Autodesk Inventor part; units mm, degrees
ref_plane "Work Plane1" through (2.381, -7.4919, 0) normal (0, 0, -1) x (0, 1, 0)
ref_plane "Work Plane2" through (2.381, -7.4919, 0) normal (1, 0, 0) x (0, 1, 0)
ref_plane "YZ Plane" through (0, 0, 0) normal (1, 0, 0) x (0, 1, 0)
sketch "Sketch1" plane through (0, 0, 0) normal (0, 0, 1) x (1, 0, 0)
  line L0 (2.381, 29.408) -> (2.381, -22.2008)
  line L1 (-18.8276, 20.7851) -> (-24.5938, 20.7851)
  line L2 (-24.5938, 20.7851) -> (-24.5938, 18.3721)
  line L3 (-24.5938, 18.3721) -> (-23.654, 18.3721)
  line L4 (-23.654, 18.3721) -> (-23.654, 16.9751)
  line L5 (-23.654, 16.9751) -> (-24.5938, 16.9751)
  line L6 (-24.5938, 16.9751) -> (-24.5938, 14.4351)
  line L7 (-24.5938, 14.4351) -> (-23.1968, 14.4351)
  line L8 (-23.1968, 14.4351) -> (-23.1968, 12.1491)
  line L9 (-23.1968, 12.1491) -> (-24.5938, 12.1491)
  line L10 (-24.5938, 12.1491) -> (-24.5938, 10.6251)
  line L11 (-24.5938, 10.6251) -> (-23.8268, 10.6251)
  line L12 (-22.2393, 9.0376) -> (-22.2393, 1.6716)
  line L13 (-23.8268, 0.0841) -> (-25.3635, 0.0841)
  line L14 (-25.3635, 0.0841) -> (-25.3635, -2.0749)
  line L15 (-25.3635, -2.0749) -> (-23.9919, -2.0749)
  line L16 (-23.9919, -2.0749) -> (-23.9919, -4.3609)
  line L17 (-23.9919, -4.3609) -> (-25.3635, -4.3609)
  line L18 (-25.3635, -4.3609) -> (-25.3635, -7.8153)
  line L19 (-25.3635, -7.8153) -> (-26.7351, -7.8153)
  line L20 (-27.7511, -8.8313) -> (-27.7511, -13.1493)
  line L21 (-26.7351, -14.1653) -> (-7.6089, -14.1653)
  line L22 (-7.6089, -14.1653) -> (-11.1851, -0.8186)
  line L23 (-11.1851, -0.8186) -> (-14.1061, -0.8186)
  line L24 (-17.2811, 2.3564) -> (-17.2811, 19.1712)
  line L25 (-17.2811, 19.1712) -> (-18.8276, 20.7851)
  arc A0 (-17.2811, 2.3564) -> (-14.1061, -0.8186) centre (-14.1061, 2.3564) ccw
  arc A1 (-22.2393, 9.0376) -> (-23.8268, 10.6251) centre (-23.8268, 9.0376) ccw
  arc A2 (-23.8268, 0.0841) -> (-22.2393, 1.6716) centre (-23.8268, 1.6716) ccw
  line L26 (-27.7511, -8.8313) -> (-26.7351, -7.8153)
  line L27 (-27.7511, -13.1493) -> (-26.7351, -14.1653)
  point P0 (-27.7511, -7.8153)
  point P1 (-27.7511, -14.1653)
  dimension "d0" = 3.175
  dimension "d1" = 1.5875
  dimension "d2" = 1.016
  dimension "d3" = 1.016
  dimension "d4" = 1.016
  dimension "d5" = 1.016
revolve "Revolution1" add sketch "Sketch1" angle 360 about axis through (2.381, 29.408, 0) along (0, -1, 0)
ref_plane "Work Plane1" through (2.381, -7.4919, 0) normal (0, 0, -1) x (0, 1, 0)
ref_plane "Work Plane2" through (2.381, -7.4919, 0) normal (1, 0, 0) x (0, 1, 0)
sketch "Sketch2" plane through (2.381, -14.1653, 0) normal (0, -1, 0) x (1, 0, 0)
  circle A0 centre (0, 0) radius 9.9898
  circle A1 centre (0, 0) radius 13.97
  line L0 (48.2112, 0) -> (-36.1584, 0)
  dimension "d7" = 27.94
sketch "Sketch3" plane through (2.381, -7.4919, 0) normal (0, 0, -1) x (0, 1, 0)
  line L0 (-10.1684, 0) -> (38.7621, 0)
  line L1 (-6.6734, -29.116) -> (-6.6734, 29.116)
  circle A0 centre (-7.7529, -13.97) radius 2.273
  line L2 (-10.1684, 0) -> (38.7621, 0)
  dimension "d9" = 1.0795
  dimension "d10" = 13.97
sweep "Sweep1" cut profiles "Sketch3" path "Sketch2" path curves A1
properties part number "Cavity-middle"
Design review of the part built by this model. Coordinates are the model's own, in mm. A direction names the side the tool comes from. Round coordinates to 2 decimals unless told otherwise and drop trailing zeros. Order: outer loops, then holes, each group sorted by start corner. A loop starts at its lowest first (then second) coordinate and runs counter-clockwise, first axis right, second up. Notation, with made-up numbers: M 36,-31 L 64,-31 A30 ccw 64,3 Z; hole C 52.25,66 d5. An arc over 180 degrees is marked long. Put each result on its own line as item: value.
Q1. Draft analysis for pull direction Y (two halves, no side actions). For faces 4 (the face through (16.5, 16.975, -22.1)), 5 (the face through (-10, -14.165, 13)), 6 (the face through (-12.534, -1.011, -23.394)), 7 (the face through (5.71, 13.28, -25.36)), state which applies: released by +Y, released by -Y, zero draft, split by the parting line, or undercut.
Reported:
face 4: undercut
face 5: released by -Y
face 6: zero draft
face 7: undercut
Q2. To check wall thickness, follow line 1 (Y direction, x = -24, z = -5); line 2 (X direction, y = 4.5, z = 0); line 3 (Y direction, x = 5.5, z = -27). State the ranges of each line that lie inside material, in increasing order.
Reported:
line 1: -14.17 to -4.36, -2.07 to 0.08, 10.63 to 12.15, 14.44 to 16.98, 18.37 to 20.79
line 2: -22.24 to -17.28, 22.04 to 27
line 3: -14.17 to -4.36, -2.07 to 0.08
Q3. Consider section A-A (y = 7.5). State the section outline as (x, z) points, and give its area (3 significant figures).
Reported:
outline: C 2.38,0 d49.24; hole C 2.38,0 d39.32
area: 690 mm²
Q4. Machinability: for faces 1 (the face through (-9.5, 20.785, 17.9)), 2 (the face through (16, -0.819, 2)), 3 (the face through (-21.5, 14.435, 9.9)), which of the approach directions +Z, -Z, +X, -X, +Y, -Y give a long, thin tool a straight path to every point of the face, cutting with its end or side? Answer none if there is none.
Reported:
face 1: +Z, -Z, +X, -X, +Y
face 2: +Y
face 3: none
Q5. Insertion check: pin 1 Ø5 at (x, y) = (11.5, -4.5) entering from +Z; pin 2 Ø17.5 at (x, z) = (-7.5, -2) entering from +Y; pin 3 Ø4 at (x, z) = (-0.5, -13.5) entering from +Y. Each pin has a flat end and moves straight along its axis. Give the tip position at first contact, or say it passes through.
Reported:
pin 1: z = 26.94
pin 2: y = 0.22
pin 3: y = -0.82
